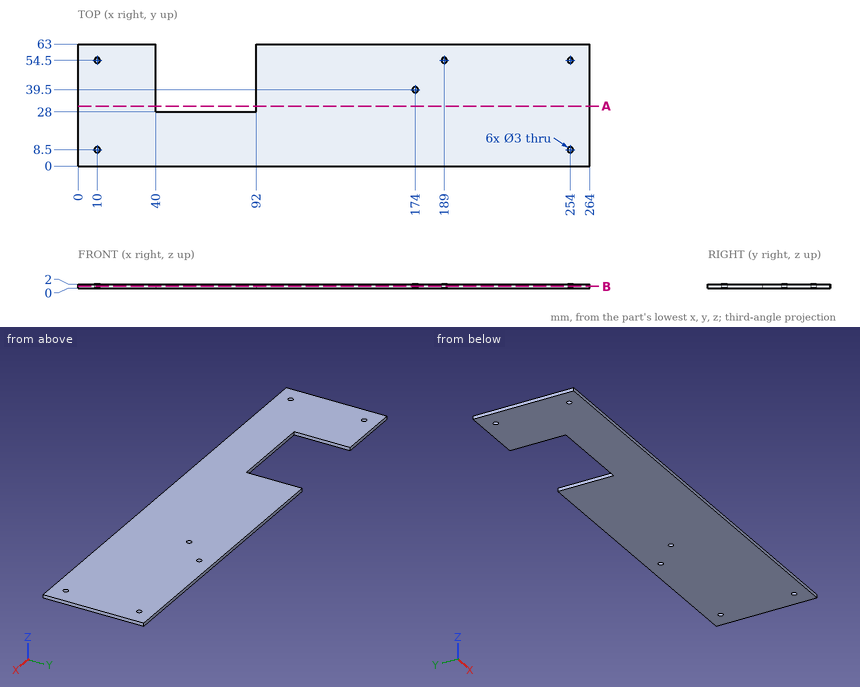
Answer from the drawing. Dimensions are ordinates in mm from the lowest x, y and z of the part. Give positions to 0.01 mm unless a question says otherwise; leave off trailing zeros. Loops run counter-clockwise (first coordinate to the right, second up) from the corner with the lowest first, then second, coordinate; pieces in that order, holes last. Notation, with made-up numbers: (-9, 38) - (-4, 38) arc R16 ccw to (-4, 47) - close; hole circle Ø6 at (18.25, 16). An arc over 180 degrees is marked (long way). Answer as a JSON object with one key per item and string values.
1. A cutting plane is placed at A-A (y = 31). Write down the section's boundary in (x, z).
Determined:
{"outline": "(0, 0) - (40, 0) - (40, 2) - (0, 2) - close; (92, 0) - (264, 0) - (264, 2) - (92, 2) - close"}
2. A cutting plane is placed at B-B (z = 0.8). Write down the section's boundary in (x, y), then the cut area to 3 significant figures.
Determined:
{"outline": "(0, 0) - (264, 0) - (264, 63) - (92, 63) - (92, 28) - (40, 28) - (40, 63) - (0, 63) - close; hole circle Ø3 at (10, 8.5); hole circle Ø3 at (10, 54.5); hole circle Ø3 at (174, 39.5); hole circle Ø3 at (189, 54.5); hole circle Ø3 at (254, 8.5); hole circle Ø3 at (254, 54.5)", "area": "14,800 mm²"}
3. Find the intervals of material crossed by L1, parallel to X at y = 54.5, z = 1.45; L2, parallel to Y at x = 254, z = 0.7; L3, parallel to X at y = 40, z = 0.2, in increasing order. Write a range as [from, to].
Determined:
{"L1": "[0, 8.5], [11.5, 40], [92, 187.5], [190.5, 252.5], [255.5, 264]", "L2": "[0, 7], [10, 53], [56, 63]", "L3": "[0, 40], [92, 172.59], [175.41, 264]"}
4. A flat-ended cylindrical pin translates along its axis: pin 1 Ø0.6 at (x, z) = (55.5, 1) entering from +Y. Find the tip coordinate at first contact, or state that the pin passes through.
Determined:
{"pin 1": "y = 28"}
